Design review of the part built by this model. Coordinates are the model's own, in mm. Face numbers are marked on the shaded views. Round coordinates to 2 decimals unless told otherwise and drop trailing zeros. Order: outer loops, then holes, each group sorted by start corner. A loop starts at its lowest first (then second) coordinate and runs counter-clockwise, first axis right, second up. Notation, with made-up numbers: (85, 63) - (139, 63) arc R18 ccw to (139, 80) - close; hole circle Ø5 at (43, -24). An arc over 180 degrees is marked (long way). Use CSV: the item, a comma, the result in double quotes.
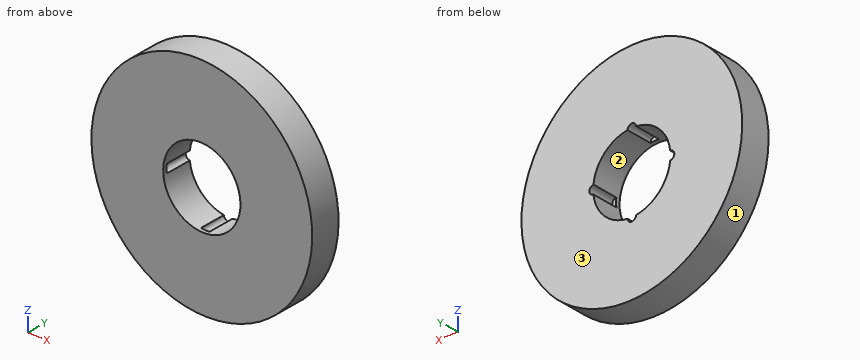
from build123d import *

# Parameters (mm, degrees)
SKETCH1_R           = 100
BOSS_EXTRUDE1_DEPTH = 27
SKETCH2_R           = 35
CUT_EXTRUDE1_DEPTH  = 144.975692393
SKETCH3_R           = 3.87281734
CUT_EXTRUDE2_DEPTH  = 23.482065
CIRPATTERN1_START   = 3.517935458
CIRPATTERN1_DEPTH   = 23.482064542


# Read off the part's stored shape, not the designer's step: CirPattern1
with BuildPart() as part:
    # Sketch1 → Boss-Extrude1 (new body)
    with BuildSketch(Plane(origin=(0, 0, 0), x_dir=(1, 0, 0), z_dir=(0, 1, 0))):
        with Locations(Location((0, 0, 0), (0, 0, 270))):
            Circle(SKETCH1_R)
    extrude(amount=BOSS_EXTRUDE1_DEPTH)

    # Sketch2 → Cut-Extrude1 (cut, through all)
    with BuildSketch(Plane(origin=(0, 0, 0), x_dir=(1, 0, 0), z_dir=(0, 1, 0))):
        with Locations(Location((0, 0, 0), (0, 0, 270))):
            Circle(SKETCH2_R)
    extrude(amount=CUT_EXTRUDE1_DEPTH, mode=Mode.SUBTRACT)

    # Sketch3 → Cut-Extrude2 (cut)
    with BuildSketch(Plane(origin=(0, 27, 0), x_dir=(1, 0, 0), z_dir=(0, 1, 0))):
        with Locations((-34.643895565, 0)):
            Circle(SKETCH3_R)
    extrude(amount=-CUT_EXTRUDE2_DEPTH, mode=Mode.SUBTRACT)

    # CirPattern1 outline → CirPattern1 (cut)
    with BuildSketch(Plane(origin=(0, 0, 0), x_dir=(1, 0, 0), z_dir=(0, 1, 0)).offset(CIRPATTERN1_START)):
        with BuildLine():
            ThreePointArc((-3.87023279, 34.7853604), (0, 35), (3.87023279, 34.7853604))
            ThreePointArc((3.87023279, 34.7853604), (0, 38.516712904), (-3.87023279, 34.7853604))
        make_face()
        with BuildLine():
            ThreePointArc((34.7853604, -3.87023279), (38.516712904, 0), (34.7853604, 3.87023279))
            ThreePointArc((34.7853604, 3.87023279), (35, 0), (34.7853604, -3.87023279))
        make_face()
        with BuildLine():
            ThreePointArc((3.87023279, -34.7853604), (0, -35), (-3.87023279, -34.7853604))
            ThreePointArc((-3.87023279, -34.7853604), (0, -38.516712904), (3.87023279, -34.7853604))
        make_face()
    extrude(amount=CIRPATTERN1_DEPTH, mode=Mode.SUBTRACT)


solid = part.part
1) To check wall thickness, follow L1, parallel to X at y = 14, z = 0; L2, parallel to Z at x = -4, y = 4.5; L3, parallel to X at y = 25.25, z = 15. State the ranges of each line that lie inside material, in increasing order. Write a range as from..to.
Data:
L1,"x = -100..-38.52, 38.52..100"
L2,"z = -99.92..-34.77, 34.77..99.92"
L3,"x = -98.87..-31.62, 31.62..98.87"
2) The part is to be moulded in two halves that separate along Z. For the marked faces 1, 2 and 3, say which applies: +Z half, -Z half, draft (parallel to the pull), parting line (faces both ways), or undercut.
Data:
face 1,"parting line"
face 2,"undercut"
face 3,"draft"
3) We need section B-B (x = 0). Give the boundary of the cut face in (y, z), then the cut area to 3 significant figures.
Data:
outline,"(0, -100) - (27, -100) - (27, -38.52) - (3.52, -38.52) - (3.52, -35) - (0, -35) - close; (0, 35) - (3.52, 35) - (3.52, 38.52) - (27, 38.52) - (27, 100) - (0, 100) - close"
area,"3,340 mm2"
4) We need section D-D (x = 30.5). Give the boundary of the cut face in (y, z).
Data:
outline,"(0, -95.24) - (27, -95.24) - (27, -17.17) - (0, -17.17) - close; (0, 17.17) - (27, 17.17) - (27, 95.24) - (0, 95.24) - close"
5) We need section C-C (z = 12). Give the boundary of the cut face in (x, y).
Data:
outline,"(-99.28, 0) - (-32.88, 0) - (-32.88, 27) - (-99.28, 27) - close; (32.88, 0) - (99.28, 0) - (99.28, 27) - (32.88, 27) - close"
6) We need section A-A (y = 14.75). Give the boundary of the cut face in (x, z).
Data:
outline,"circle Ø200 at (0, 0); hole (-34.79, -3.87) arc R35 ccw to (-3.87, -34.79) arc R3.87 ccw to (3.87, -34.79) arc R35 ccw to (34.79, -3.87) arc R3.87 ccw to (34.79, 3.87) arc R35 ccw to (3.87, 34.79) arc R3.87 ccw to (-3.87, 34.79) arc R35 ccw to (-34.79, 3.87) arc R3.87 ccw to start"
7) Insertion check: pin 1 Ø1.9 at (x, z) = (36.5, -1) entering from +Y; pin 2 Ø2 at (x, y) = (-48.5, 14) entering from -Z; pin 3 Ø10 at (y, z) = (14, -12) entering from +X. Each pin has a flat end and moves straight along its axis. Give the tip position at first contact, or say it passes through.
Data:
pin 1,"stops at y = 3.52"
pin 2,"stops at z = -88"
pin 3,"stops at x = 99.75"
